Work out the finished part from the listing and answer in its coordinate system (mm). A direction names the side the tool comes from. Give positions to 0.01 mm unless a question says otherwise; leave off trailing zeros. Order: outer loops, then holes, each group sorted by start corner. A loop starts at its lowest first (then second) coordinate and runs counter-clockwise, first axis right, second up. Notation, with made-up numbers: (56.5, 26.25) -> (77.5, 26.25) arc R21 ccw to (77.5, 33.25) -> close; hole circle Ø8 at (56, 31). An arc over 180 degrees is marked (long way). Answer as CSV lines item,"result". Start each with the question number.
1. A cutting plane is placed at C-C (x = -271.5). Give the vertices of the cut face in (y, z) (3 decimals), then the cut area to 3 significant figures.
2. A cutting plane is placed at A-A (x = -233.5). Give the vertices of the cut face in (y, z).
3. For faces 1 (the cylindrical face through (-215.381, 151.915, 2.465)), 2 (the flat face through (-272, 160, 21)), 3 (the cylindrical face through (-221, 123, 70)), 4 (the flat face through (-203.49, 135, 2)), 5 (the flat face through (-170, 135, 61)), determine the directions among +Z, -Z, +X, -X, +Y, -Y from which every point of the face is accessible in a straight line to the end or side of a thin tool.
4. For a pull along X with two mould halves and no side action, classify faces 6 (the cylindrical face through (-245.23, 148.5, 2.46)), 7 (the cylindrical face through (-299.14, 159.1, 27.12)), 8 (the flat face through (-270, 135, 34)), 9 (the flat face through (-237, 135, 5)) as released by +X, released by -X, zero draft, split by the parting line, or undercut.
5. Flat-ended cylindrical pins translate along their axes: pin 1 (1.5 mm diameter, centred on y = 144.5, z = 1.5, fed in from +X); pin 2 (4 mm diameter, centred on x = -283.5, z = 68, fed in from -Y); pin 3 (8 mm diameter, centred on x = -220, y = 120, fed in from -Z). Find the tip coordinate at first contact, or state that the pin passes through.
6. A cutting plane is placed at B-B (z = 13.5). Give the vertices of the cut face in (x, y), then the cut area to 3 significant figures.
7. A cutting plane is placed at D-D (z = 49). Give the vertices of the cut face in (x, y).
8. Find the intervals of material crossed by L1, parallel to Y at x = -220, z = 3.1; L2, parallel to X at y = 114, z = 55; L3, parallel to Z at x = -266, y = 132, in increasing order.
Autodesk Fusion 360 part; units mm, degrees
sketch "Sketch3" plane through (0, 0, 0) normal (0, 0, 1) x (1, 0, 0)
  circle A0 centre (-250, 150) radius 5
  circle A1 centre (-220, 150) radius 5
  circle A2 centre (-250, 120) radius 5
  circle A3 centre (-220, 120) radius 5
  line L0 (-270, 160) -> (-203.4896, 160)
  line L1 (-203.4896, 160) -> (-203.4896, 110)
  line L2 (-203.4896, 110) -> (-270, 110)
  line L3 (-270, 110) -> (-270, 160)
  line L4 (-270, 160) -> (-300, 160)
  line L5 (-300, 160) -> (-300, 110)
  line L6 (-300, 110) -> (-270, 110)
  line L7 (-270, 110) -> (-270, 160)
  dimension "d13" = 10
  dimension "d14" = 10
  dimension "d15" = 10
  dimension "d16" = 10
extrude "Extrude1" add sketch "Sketch3" along normal blind 5 contours L0 L1 L2 L3 L7
extrude "Extrude2" add sketch "Sketch3" along normal blind 80 contours L3 L4 L5 L6 L7
sketch "Sketch6" plane through (-270, 0, 0) normal (1, 0, 0) x (0, 1, 0)
  line L0 (110, 5) -> (160, 5)
  line L1 (160, 5) -> (160, 80)
  line L2 (160, 80) -> (110, 80)
  line L3 (110, 80) -> (110, 0)
  circle A0 centre (135, 61) radius 15
  line L4 (110, 0) -> (110, 0)
  line L5 (110, 0) -> (110, 5)
  dimension "d6" = 30
extrude "Extrude3" add sketch "Sketch6" along normal blind 100 contours A0
fillet "Fillet1" radius 25 2 edges at (-285, 160, 80) (-285, 110, 80)
fillet "Fillet3" radius 3 5 edges at (-203.4896, 160, 2.5) (-203.4896, 110, 2.5) (-300, 110, 27.5) (-300, 135, 80) (-300, 160, 27.5)
Answer sheet:
1,outline,"(110, 0) -> (160, 0) -> (160, 55.005) arc R24.995 ccw to (135.005, 80) -> (134.995, 80) arc R24.995 ccw to (110, 55.005) -> close"
1,area,"3,730 mm^2"
2,outline,"(110, 0) -> (160, 0) -> (160, 5) -> (110, 5) -> close; circle Ø30 at (135, 61)"
3,face 1,"-Z"
3,face 2,"+Z, -Z, +X, -X, +Y"
3,face 3,"+X"
3,face 4,"-Z, +X, +Y, -Y"
3,face 5,"+Z, -Z, +X, +Y, -Y"
4,face 6,"undercut"
4,face 7,"released by -X"
4,face 8,"released by +X"
4,face 9,"zero draft"
5,pin 1,"stops at x = -203.49"
5,pin 2,"stops at y = 112.55"
5,pin 3,"stops at z = 50.8"
6,outline,"(-300, 113) arc R3 ccw to (-297, 110) -> (-270, 110) -> (-270, 160) -> (-297, 160) arc R3 ccw to (-300, 157) -> close"
6,area,"1,500 mm^2"
7,outline,"(-300, 113) arc R3 ccw to (-297, 110) -> (-270, 110) -> (-270, 126) -> (-170, 126) -> (-170, 144) -> (-270, 144) -> (-270, 160) -> (-297, 160) arc R3 ccw to (-300, 157) -> close"
8,L1,"y = 110 to 115, 125 to 145, 155 to 160"
8,L2,"x = -300 to -270"
8,L3,"z = 0 to 5, 46.3 to 75.7"
